The listing builds one solid part. Answer for the finished solid, in the listing's coordinates (mm). A direction names the side the tool comes from. Give positions to 0.01 mm unless a question says otherwise; leave off trailing zeros. Order: outer loops, then holes, each group sorted by start corner. A loop starts at its lowest first (then second) coordinate and runs counter-clockwise, first axis right, second up. Notation, with made-up numbers: (-18.75, -11.75) - (32.25, -11.75) arc R10 ccw to (32.25, -4.75) - close; hole circle Ø5 at (41.25, -32). An arc over 180 degrees is marked (long way). Write each question's results on one line, items separated by ' | '. Start each with the question number.
1. Determine the mould class of faces 5 (the face through (7, -7, 140.729)), 6 (the face through (-1, -1, -83.4)), 7 (the face through (0.363, -48.034, -0.056)) for opening direction Z: released by +Z, released by -Z, zero draft, split by the parting line, or undercut.
2. Section C-C (y = 0) is taken. State how many separate pieces and enclosed holes the cut face has, and give its area (3 significant figures).
3. Flat-ended cylindrical pins translate along their axes: pin 1 (9 mm diameter, centred on x = 35.92, y = -35.92, fed in from +Z); pin 2 (12 mm diameter, centred on y = 38, z = 58.5, fed in from -X); pin 3 (12 mm diameter, centred on x = -9.5, y = -31, fed in from +Z); pin 4 (3.5 mm diameter, centred on x = -12.84, y = -4.17, fed in from +Z). Find the tip coordinate at first contact, or state that the pin passes through.
4. Section B-B (z = 55) is taken. Give the vertices of the cut face in (x, y), and give its area (3 significant figures).
5. Section A-A (y = -50.8) is taken. Give the vertices of the cut face in (x, z).
6. Which of the six approach directions +Z, -Z, +X, -X, +Y, -Y give full straight-line access (tool end or side, diameter ignored) to faces 1 (the face through (0, 0, 148.816)), 2 (the face through (20.765, 39.923, -43.144)), 3 (the face through (7, -7, 143.431)), 4 (the face through (21.199, 6.676, 132.016))?
7. Section D-D (z = -48.5) is taken. Give the vertices of the cut face in (x, y).
8. Find the intervals of material crossed by L1, parallel to Z at x = 10.5, y = -2; L2, parallel to Y at x = 50.8, z = 1.25; L3, parallel to Z at x = 24.5, y = 25, in increasing order.
from build123d import *

# Parameters (mm, degrees)
SKETCH1_R          = 57.15
EXTRUDE1_DEPTH     = 4
SKETCH3_R          = 7.5
EXTRUDE2_DEPTH     = 12.166
SKETCH4_R          = 36.5
EXTRUDE3_DEPTH     = 107.24
SKETCH5_R          = 22.225
EXTRUDE4_DEPTH     = 17.3228
SKETCH6_R          = 9.525
EXTRUDE5_DEPTH     = 2.702052
SKETCH7_R          = 16.5
EXTRUDE6_DEPTH     = 5.3848
SKETCH8_R          = 1.6
CUT_EXTRUDE1_DEPTH = 5.3848
SKETCH10_R         = 2.79
CUT_EXTRUDE2_DEPTH = 8
SKETCH11_R         = 45
EXTRUDE7_DEPTH     = 79.4
FILLET1_R          = 5


with BuildPart() as part:
    # Sketch1 → Extrude1 (new body, symmetric)
    with BuildSketch(Plane.XY):
        Circle(SKETCH1_R)
    extrude(amount=EXTRUDE1_DEPTH, both=True)

    # Sketch3 → Extrude2 (add)
    with BuildSketch(Plane.XY.offset(4)):
        Circle(SKETCH3_R)
    extrude(amount=EXTRUDE2_DEPTH)

    # Sketch4 → Extrude3 (add)
    with BuildSketch(Plane.XY.offset(16.166)):
        Circle(SKETCH4_R)
    extrude(amount=EXTRUDE3_DEPTH)

    # Sketch5 → Extrude4 (add)
    with BuildSketch(Plane.XY.offset(123.406)):
        Circle(SKETCH5_R)
    extrude(amount=EXTRUDE4_DEPTH)

    # Sketch6 → Extrude5 (add)
    with BuildSketch(Plane.XY.offset(140.7288)):
        Circle(SKETCH6_R)
    extrude(amount=EXTRUDE5_DEPTH)

    # Sketch7 → Extrude6 (add)
    with BuildSketch(Plane.XY.offset(143.430852)):
        Circle(SKETCH7_R)
    extrude(amount=EXTRUDE6_DEPTH)

    # Sketch8 → Cut-Extrude1 (cut)
    with BuildSketch(Plane.XY.offset(148.815652)):
        with Locations((-7.935100906, 10.921729424)):
            Circle(SKETCH8_R)
        with Locations((7.935100906, 10.921729424)):
            Circle(SKETCH8_R)
        with Locations((12.83926297, -4.171729424)):
            Circle(SKETCH8_R)
        with Locations((0, -13.5)):
            Circle(SKETCH8_R)
        with Locations((-12.83926297, -4.171729424)):
            Circle(SKETCH8_R)
    extrude(amount=-CUT_EXTRUDE1_DEPTH, mode=Mode.SUBTRACT)

    # Sketch10 → Cut-Extrude2 (cut)
    with BuildSketch(Plane(origin=(0, 0, -4), x_dir=(-1, 0, 0), z_dir=(0, 0, -1))):
        with Locations((0, 50.8)):
            Circle(SKETCH10_R)
        with Locations((35.921024484, 35.921024484)):
            Circle(SKETCH10_R)
        with Locations((50.8, 0)):
            Circle(SKETCH10_R)
        with Locations((35.921024484, -35.921024484)):
            Circle(SKETCH10_R)
        with Locations((0, -50.8)):
            Circle(SKETCH10_R)
        with Locations((-35.921024484, -35.921024484)):
            Circle(SKETCH10_R)
        with Locations((-50.8, 0)):
            Circle(SKETCH10_R)
        with Locations((-35.921024484, 35.921024484)):
            Circle(SKETCH10_R)
    extrude(amount=-CUT_EXTRUDE2_DEPTH, mode=Mode.SUBTRACT)

    # Sketch11 → Extrude7 (add)
    with BuildSketch(Plane(origin=(0, 0, -4), x_dir=(-1, 0, 0), z_dir=(0, 0, -1))):
        with Locations(Location((0, 0, 0), (0, 0, 180))):  # turned: the seam where the file's is
            Circle(SKETCH11_R)
    extrude(amount=EXTRUDE7_DEPTH)

    # Fillet1
    fillet1_edges = [part.edges().sort_by_distance(p)[0] for p in [
        (-36.5, 0, 123.406),
        (-22.225, 0, 123.406),
        (-22.225, 0, 140.7288),
        (-36.5, 0, 16.166),
    ]]
    fillet(fillet1_edges, radius=FILLET1_R)


solid = part.part
Reported:
1) face 5: undercut | face 6: released by -Z | face 7: zero draft
2) separate pieces: 3 | enclosed holes: 0 | area: 17,000 mm²
3) pin 1: z = 4 | pin 2: x = -17.56 | pin 3: z = 123.47 | pin 4: z = 148.82
4) outline: circle Ø73 at (0, 0) | area: 4,190 mm²
5) outline: (-26.18, -4) - (-2.79, -4) - (-2.79, 4) - (-26.18, 4) - close; (2.79, -4) - (26.18, -4) - (26.18, 4) - (2.79, 4) - close
6) face 1: +Z, +X, -X, +Y, -Y | face 2: -Z | face 3: none | face 4: +Z
7) outline: circle Ø90 at (0, 0)
8) L1: -83.4 to 4, 16.17 to 140.73, 143.43 to 148.82 | L2: -26.18 to -2.79, 2.79 to 26.18 | L3: -83.4 to 4, 17.6 to 121.97
